```python
from build123d import *

# Parameters (mm, degrees)
F0_R     = 25
F1_DEPTH = 50
F2_T     = -2
F3_R     = 22.120492
F4_DEPTH = 25


with BuildPart() as f1:
    # F0 (on Top) → F1 (new body)
    with BuildSketch(Plane.XY):
        Circle(F0_R)
    extrude(amount=F1_DEPTH)

    # F2
    f2_openings = [f1.faces().sort_by_distance(p)[0] for p in [
        (0, 0, 0),
    ]]
    offset(amount=F2_T, openings=f2_openings)

    # F3 (on face) → F4 (cut)
    with BuildSketch(Plane(origin=(0, 0, 48), x_dir=(1, 0, 0), z_dir=(0, 0, -1))):
        Circle(F3_R)
    extrude(amount=-F4_DEPTH, mode=Mode.SUBTRACT)


solid = f1.part
```
The model under review builds one solid part; all positions refer to its coordinate system, in mm. Round coordinates to 2 decimals unless told otherwise and drop trailing zeros. Loops run counter-clockwise (first coordinate to the right, second up) from the corner with the lowest first, then second, coordinate; pieces in that order, holes last. Notation, with made-up numbers: (-2, 1.5) - (55, 1.5) arc R22 cw to (55, 19.5) - close; hole circle Ø6 at (48, 3). An arc over 180 degrees is marked (long way). Write each question's results on one line, items separated by ' | '. Start each with the question number.
Q1. Insertion check: P1, Ø10, axis at x = 8.5, y = -9.5, coming from the +Z side; P2, Ø5, axis at x = -1, z = 10, coming from the +Y side; P3, Ø10, axis at y = 6.5, z = 8.5, coming from the +X side; P4, Ø1, axis at x = 17.5, z = 21.5, coming from the -Y side. Each pin has a flat end and moves straight along its axis. Give the tip position at first contact, or say it passes through.
Q2. Wall thickness on line 1 along Y through (x, z) = (0, 48.5); line 2 along X through (y, z) = (-14, 30); line 3 along Y through (x, z) = (0, 34.5): over which ranges is each line inside the solid? List them lowest first. Write a range as [from, to].
Q3. Take a section at A-A on x = 0. Give the boundary of the cut face in (y, z).
Q4. Take a section at C-C on z = 11. Give the boundary of the cut face in (x, y), plus the area to 3 significant figures.
Q5. Draft analysis for pull direction Y (two halves, no side actions). For faces 1 (the cylindrical face through (-2.994, 22.804, 23.664)), 2 (the cylindrical face through (23.846, 7.509, 24.65)), 3 (the flat face through (22.1, -7.3, 0)), 4 (the flat face through (-12, 19, 48)), state which applies: pulls with the +Y half, pulls with the -Y half, needs draft (parallel to the pull), parting line crosses it, or undercut.
Data:
1) P1: passes through | P2: stops at y = 25 | P3: stops at x = 24.95 | P4: stops at y = -18.33
2) line 1: y = [-25, -22.12], [22.12, 25] | line 2: x = [-20.71, -18.25], [18.25, 20.71] | line 3: y = [-25, -23], [23, 25]
3) outline: (-25, 0) - (-23, 0) - (-23, 48) - (-22.12, 48) - (-22.12, 50) - (-25, 50) - close; (22.12, 48) - (23, 48) - (23, 0) - (25, 0) - (25, 50) - (22.12, 50) - close
4) outline: circle Ø50 at (0, 0); hole circle Ø46 at (0, 0) | area: 302 mm²
5) face 1: undercut | face 2: parting line crosses it | face 3: needs draft | face 4: undercut
